Part print with two shaded views. Sizes in mm from the minimum x, y, z corner. A direction names the side the tool comes from. Coordinates: 2 decimals unless noted, no trailing zeros. Loops run counter-clockwise (first coordinate to the right, second up) from the corner with the lowest first, then second, coordinate; pieces in that order, holes last.
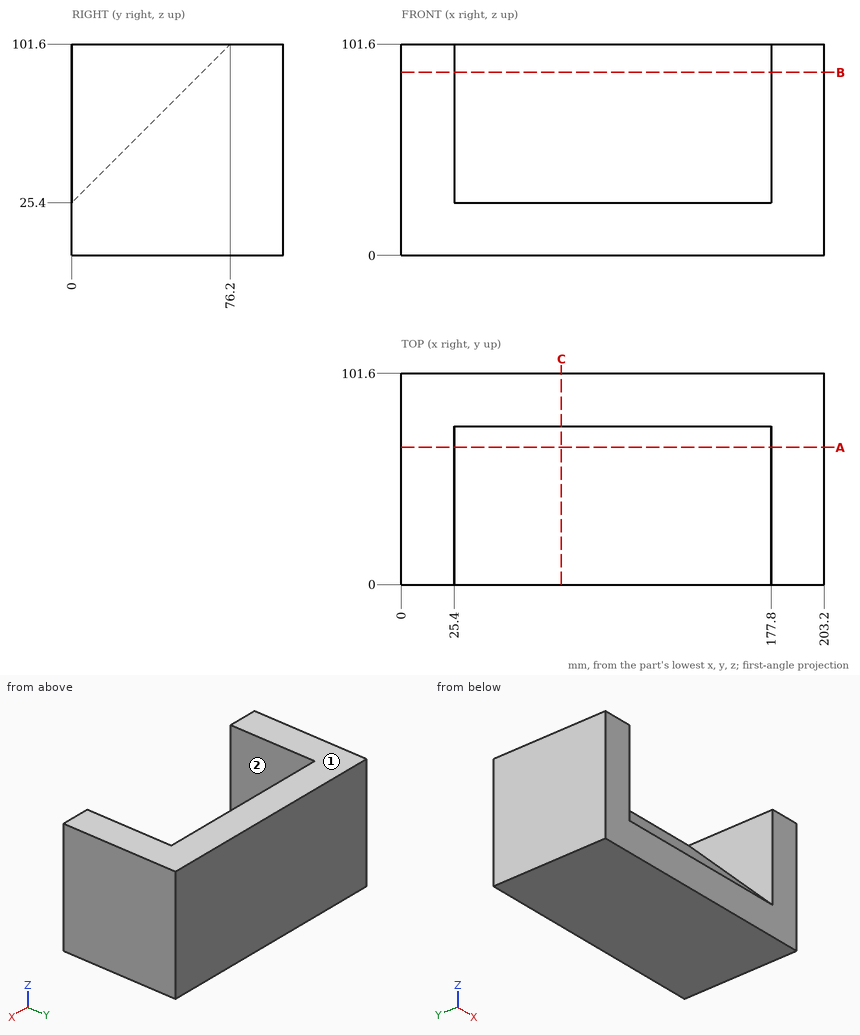
Q1. Which spindle directions (+Z, -Z, +X, -X, +Y, -Y) get a long thin tool onto all of the face, cutting with end or side? Do the marked faces 1 and 2. Say none if no direction does.
Answers:
face 1: +Z, +X, -X, +Y, -Y
face 2: +Z, -Y
Q2. Drill centre lines: line 1 (X direction, y = 24, z = 75.5); line 2 (Y direction, x = 123, z = 44); line 3 (Y direction, x = 154, z = 31.5). Where is each one in solid material? Low to high.
Answers:
line 1: x = 0 to 25.4, 177.8 to 203.2
line 2: y = 18.6 to 101.6
line 3: y = 6.1 to 101.6
Q3. Slice it at C-C (x = 77). List the corners of the cut face in (y, z), and give its area (3 significant figures).
Answers:
outline: (0, 0) - (101.6, 0) - (101.6, 101.6) - (76.2, 101.6) - (0, 25.4) - close
area: 7,420 mm2
Q4. Slice it at B-B (z = 88). List the corners of the cut face in (x, y).
Answers:
outline: (0, 0) - (25.4, 0) - (25.4, 62.6) - (177.8, 62.6) - (177.8, 0) - (203.2, 0) - (203.2, 101.6) - (0, 101.6) - close
Q5. Slice it at A-A (y = 66). List the corners of the cut face in (x, z), and give its area (3 significant figures).
Answers:
outline: (0, 0) - (203.2, 0) - (203.2, 101.6) - (177.8, 101.6) - (177.8, 91.4) - (25.4, 91.4) - (25.4, 101.6) - (0, 101.6) - close
area: 19,100 mm2
